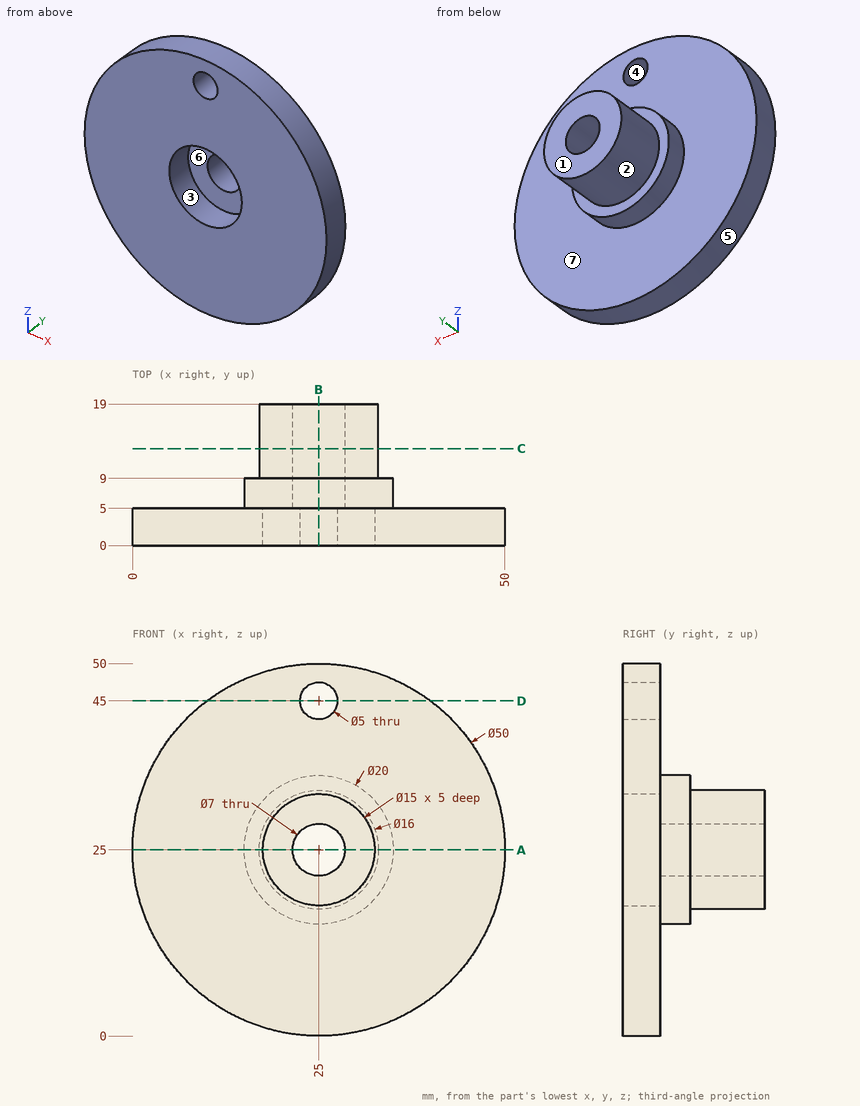
Design review of the part shown in the three views and the two pictorial views. Dimensions are in mm from the part's minimum x, y and z. A direction names the side the tool comes from. Round coordinates to 2 decimals unless told otherwise and drop trailing zeros. Write each loop counter-clockwise with the first axis right and the second up, starting at its lowest first coordinate (ties: lowest second). Pieces come first, ordered by that corner, then holes. Notation, with made-up numbers: (-21, 71) -> (-9, 71) arc R7 ccw to (-9, 78) -> close; hole circle Ø2 at (-36, 73). An arc over 180 degrees is marked (long way). One line per question, with ' | ' between items. Start each with the question number.
1) Add section A-A (z = 25). Write out the cut boundary in (x, y), and give its area (3 significant figures).
2) Add section C-C (y = 13). Write out the cut boundary in (x, z), and give its area (3 significant figures).
3) Add section B-B (x = 25). Write out the cut boundary in (y, z).
4) For pin 1 Ø3 at (x, z) = (25, 45) entering from -Y; pin 2 Ø2 at (x, y) = (32.5, 14.5) entering from -Z; pin 3 Ø8 at (x, z) = (37.5, 16) entering from +Y; pin 4 Ø17 at (x, z) = (25, 25) entering from -Y, all flat-tipped, find the tip position at first contact; note any pin that passes through.
5) Machinability: for the marked faces 5, 6 and 7, which of the approach directions +Z, -Z, +X, -X, +Y, -Y give a long, thin tool a straight path to every point of the face, cutting with its end or side? Answer none if there is none.
6) Wall thickness on line 1 along Z through (x, y) = (25, 1); line 2 along X through (y, z) = (10.5, 25): over which ranges is each line inside the solid? List them lowest first.
7) Add section D-D (z = 45). Write out the cut boundary in (x, y).
8) Mouldability with a two-part tool opening along X and no side actions: class the marked faces 1, 2, 3 and 4 as +X half, -X half, draft (parallel to the pull), parting line (faces both ways), or undercut.
Reported:
1) outline: (0, 0) -> (17.5, 0) -> (17.5, 5) -> (21.5, 5) -> (21.5, 19) -> (17, 19) -> (17, 9) -> (15, 9) -> (15, 5) -> (0, 5) -> close; (28.5, 5) -> (32.5, 5) -> (32.5, 0) -> (50, 0) -> (50, 5) -> (35, 5) -> (35, 9) -> (33, 9) -> (33, 19) -> (28.5, 19) -> close | area: 317 mm²
2) outline: circle Ø16 at (25, 25); hole circle Ø7 at (25, 25) | area: 163 mm²
3) outline: (0, 0) -> (5, 0) -> (5, 15) -> (9, 15) -> (9, 17) -> (19, 17) -> (19, 21.5) -> (5, 21.5) -> (5, 17.5) -> (0, 17.5) -> close; (0, 32.5) -> (5, 32.5) -> (5, 28.5) -> (19, 28.5) -> (19, 33) -> (9, 33) -> (9, 35) -> (5, 35) -> (5, 42.5) -> (0, 42.5) -> close; (0, 47.5) -> (5, 47.5) -> (5, 50) -> (0, 50) -> close
4) pin 1: passes through | pin 2: stops at z = 20.34 | pin 3: stops at y = 5 | pin 4: stops at y = 0
5) face 5: +Y, -Y | face 6: -Y | face 7: +Y
6) line 1: z = 0 to 17.5, 32.5 to 42.5, 47.5 to 50 | line 2: x = 17 to 21.5, 28.5 to 33
7) outline: (10, 0) -> (22.5, 0) -> (22.5, 5) -> (10, 5) -> close; (27.5, 0) -> (40, 0) -> (40, 5) -> (27.5, 5) -> close
8) face 1: draft | face 2: parting line | face 3: undercut | face 4: undercut
